from build123d import *

# Parameters (mm, degrees)
F0_W     = 39.9999970493
F0_H     = 20
F1_DEPTH = 20
F3_D     = 4
F5_D     = 6
F6_R     = 9.99999
F7_R     = 9.99999


# Not quite as in the source:
# - a fillet or chamfer is up to 0.001 mm smaller than in the source, because OpenCascade refuses the exact size


with BuildPart() as f1:
    # F0 (on Top) → F1 (new body)
    with BuildSketch(Plane.XY):
        with Locations((19.9999985246, 10)):
            Rectangle(F0_W, F0_H)
    extrude(amount=F1_DEPTH)

    # F3 (through all)
    with Locations(Plane.XY.offset(20)):
        with Locations((30.0000011921, 10)):
            Hole(F3_D / 2)

    # F5 (through all)
    with Locations(Plane.XZ):
        with Locations((10, 10)):
            Hole(F5_D / 2)

    # F6 (radius 10 in the source; OpenCascade refuses exactly that, so slightly less here)
    f6_edges = [f1.edges().sort_by_distance(p)[0] for p in [
        (39.999997, 0, 10),
        (39.999997, 20, 10),
    ]]
    fillet(f6_edges, radius=F6_R)

    # F7 (radius 10 in the source; OpenCascade refuses exactly that, so slightly less here)
    f7_edges = [f1.edges().sort_by_distance(p)[0] for p in [
        (0, 10, 0),
        (0, 10, 20),
    ]]
    fillet(f7_edges, radius=F7_R)


solid = f1.part
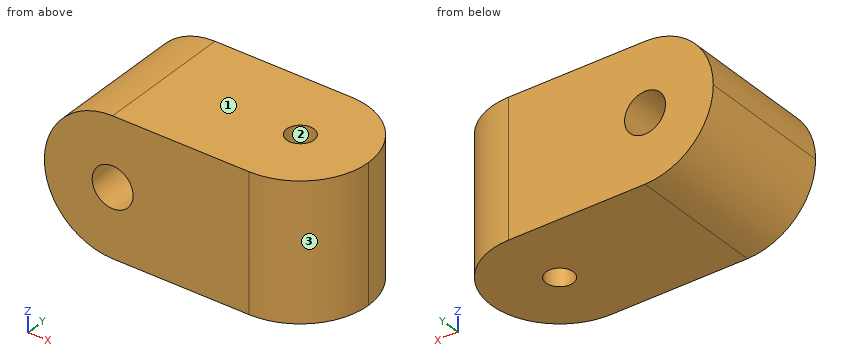
Source: CAD feature listing. Evaluate the final solid. Frame: model axes, mm. Face numbers are marked on the shaded views. Round coordinates to 2 decimals unless told otherwise and drop trailing zeros. Loops run counter-clockwise (first coordinate to the right, second up) from the corner with the lowest first, then second, coordinate; pieces in that order, holes last. Notation, with made-up numbers: (0.5, 88.25) - (8.5, 88.25) arc R29 ccw to (8.5, 108.25) - close; hole circle Ø1 at (19.5, 68.5). An arc over 180 degrees is marked (long way). Write item = value, one per line. Start each with the question number.
Item 1: Material intervals for line 1 (Z direction, x = 10, y = 4.25); line 2 (Y direction, x = 30, z = 5.75); line 3 (Z direction, x = 3.5, y = 1.75), sorted ascending.
Item 2: First-contact query: pin 1 Ø1 at (x, y) = (5, 7.5) entering from -Z; pin 2 Ø3.5 at (x, z) = (10, 10) entering from +Y. Flat tips, straight axial feed; report the tip coordinate or a pass-through.
Item 3: Section query A-A on z = 11.75. Count the separate pieces of the cut face and the enclosed holes in it, plus the area to 3 significant figures.
Item 4: Section query D-D on x = 12. Output: boundary loops of the cut face in (y, z), plus the area to 3 significant figures.
Item 5: Mould query, pull axis Y, two halves, no side actions, for the marked faces 1, 2 and 3. Classes: released by +Y, released by -Y, zero draft, split by the parting line, or undercut.
Results list:
q1.line_1 = 0 to 7, 13 to 20
q1.line_2 = 0 to 8, 12 to 20
q1.line_3 = 2.4 to 17.6
q2.pin_1 = 1.07
q2.pin_2 = through
q3.separate_pieces = 2
q3.enclosed_holes = 1
q3.area = 644 mm²
q4.outline = (0, 0) - (20, 0) - (20, 7.76) - (0, 7.76) - close; (0, 12.24) - (20, 12.24) - (20, 20) - (0, 20) - close
q4.area = 311 mm²
q5.face_1 = zero draft
q5.face_2 = undercut
q5.face_3 = released by -Y
